The model under review builds one solid part; all positions refer to its coordinate system, in mm. A direction names the side the tool comes from. Coordinates: 2 decimals unless noted, no trailing zeros. Loops run counter-clockwise (first coordinate to the right, second up) from the corner with the lowest first, then second, coordinate; pieces in that order, holes last. Notation, with made-up numbers: (-31, 31) - (-13, 31) arc R8 cw to (-13, 40) - close; hole circle Ø2 at (75, 68). An arc over 180 degrees is marked (long way). One line per item, written item: value. Start each with the question number.
1. We need section A-A, the plane z = 33. Give the boundary of the cut face in (x, y), then the cut area to 3 significant figures.
2. Mouldability with a two-part tool opening along Y and no side actions: class faces 4 (the face through (0, 0, 0)), 5 (the face through (3, 1, 28)), 6 (the face through (-13.887, -10.648, 14.79)) as +Y half, -Y half, draft (parallel to the pull), parting line (faces both ways), or undercut.
3. To check wall thickness, follow line 1 (Y direction, x = 0, z = 29.1); line 2 (Y direction, x = 0, z = 36); line 3 (Z direction, x = 3.5, y = 12.5). State the ranges of each line that lie inside material, in increasing order.
4. We need section C-C, the plane z = 24. Give the boundary of the cut face in (x, y).
5. Insertion check: P1, Ø4, axis at x = -11.5, y = -10.5, coming from the -Z side; P2, Ø4, axis at x = 2, y = -11, coming from the +Z side; P3, Ø1.5, axis at y = -4.5, z = 32.5, coming from the -X side; P4, Ø1.5, axis at y = -7.5, z = 16.5, coming from the -X side. Each pin has a flat end and moves straight along its axis. Give the tip position at first contact, or say it passes through.
6. We need section D-D, the plane y = -5. Give the boundary of the cut face in (x, z) (1 decimal), then the cut area to 3 significant figures.
7. For faces 1 (the face through (2, 0, 46)), 2 (the face through (-3, 0, 38)), 3 (the face through (0, 0, 50)), list the 3-axis set-ups (+Z, -Z, +X, -X, +Y, -Y) from which the entire face can be reached by the end or side of a thin tool; tool diameter is ignored.
8. We need section B-B, the plane x = 0. Give the boundary of the cut face in (y, z), then the cut area to 3 significant figures.
from build123d import *

# Parameters (mm, degrees)
SKETCH_1_R          = 17.5
EXTRUDE_1_DEPTH     = 30
SKETCH_2_R          = 8
EXTRUDE_2_DEPTH     = 10
CUT_EXTRUDE_START   = -2
SKETCH_3_R          = 8.5
SKETCH_3_R_2        = 8
CUT_EXTRUDE_1_DEPTH = 2
SKETCH_4_R          = 3
EXTRUDE_3_DEPTH     = 10
CUT_EXTRUDE_START_2 = -12
SKETCH_5_R          = 3.5
SKETCH_5_R_2        = 3
CUT_EXTRUDE_2_DEPTH = 12
FILLET_1_R          = 1
SKETCH_6_W          = 2.555325261
SKETCH_6_H          = 9.362978713
CUT_EXTRUDE_3_DEPTH = 8


with BuildPart() as part:
    # 草图1 → 凸台-拉伸1 (new body)
    with BuildSketch(Plane.XY):
        Circle(SKETCH_1_R)
    extrude(amount=EXTRUDE_1_DEPTH)

    # 草图2 → 凸台-拉伸2 (add)
    with BuildSketch(Plane.XY.offset(30)):
        Circle(SKETCH_2_R)
    extrude(amount=EXTRUDE_2_DEPTH)

    # 草图3 → 切除-拉伸1 (cut)
    with BuildSketch(Plane.XY.offset(30).offset(CUT_EXTRUDE_START)):
        Circle(SKETCH_3_R)
        Circle(SKETCH_3_R_2, mode=Mode.SUBTRACT)
    extrude(amount=CUT_EXTRUDE_1_DEPTH, mode=Mode.SUBTRACT)

    # 草图4 → 凸台-拉伸3 (add)
    with BuildSketch(Plane.XY.offset(40)):
        Circle(SKETCH_4_R)
    extrude(amount=EXTRUDE_3_DEPTH)

    # 草图5 → 切除-拉伸2 (cut)
    with BuildSketch(Plane.XY.offset(40).offset(CUT_EXTRUDE_START_2)):
        Circle(SKETCH_5_R)
        Circle(SKETCH_5_R_2, mode=Mode.SUBTRACT)
    extrude(amount=CUT_EXTRUDE_2_DEPTH, mode=Mode.SUBTRACT)

    # 圆角1
    fillet_1_edges = [part.edges().sort_by_distance(p)[0] for p in [
        (-3, 0, 50),
    ]]
    fillet(fillet_1_edges, radius=FILLET_1_R)

    # 草图6 → 切除-拉伸3 (cut)
    with BuildSketch(Plane.XY.offset(50)):
        with Locations((3.277662631, -1.004075507)):
            Rectangle(SKETCH_6_W, SKETCH_6_H)
    extrude(amount=-CUT_EXTRUDE_3_DEPTH, mode=Mode.SUBTRACT)


solid = part.part
Findings below:
1. outline: circle Ø16 at (0, 0); circle Ø6 at (0, 0); hole circle Ø7 at (0, 0)
1. area: 191 mm2
2. face 4: draft
2. face 5: undercut
2. face 6: parting line
3. line 1: -17.5 to -8.5, -8 to -3.5, -3 to 3, 3.5 to 8, 8.5 to 17.5
3. line 2: -8 to -3.5, -3 to 3, 3.5 to 8
3. line 3: 0 to 30
4. outline: circle Ø35 at (0, 0)
5. P1: z = 0
5. P2: z = 30
5. P3: x = -7.07
5. P4: x = -16.15
6. outline: (-16.8, 0) - (16.8, 0) - (16.8, 30) - (6.9, 30) - (6.9, 28) - (6.2, 28) - (6.2, 40) - (-6.2, 40) - (-6.2, 28) - (-6.9, 28) - (-6.9, 30) - (-16.8, 30) - close
6. area: 1,130 mm2
7. face 1: +Z, +X, +Y, -Y
7. face 2: +Z
7. face 3: +Z, +X, -X, +Y, -Y
8. outline: (-17.5, 0) - (17.5, 0) - (17.5, 30) - (8.5, 30) - (8.5, 28) - (8, 28) - (8, 40) - (3.5, 40) - (3.5, 28) - (3, 28) - (3, 49) arc R1 ccw to (2, 50) - (-2, 50) arc R1 ccw to (-3, 49) - (-3, 28) - (-3.5, 28) - (-3.5, 40) - (-8, 40) - (-8, 28) - (-8.5, 28) - (-8.5, 30) - (-17.5, 30) - close
8. area: 1,260 mm2
